Check sheet for the drawn part. Datum: minimum x, y, z corner. Units: mm. A direction names the side the tool comes from. Give positions to 0.01 mm unless a question says otherwise; leave off trailing zeros. Loops run counter-clockwise (first coordinate to the right, second up) from the corner with the lowest first, then second, coordinate; pieces in that order, holes last.
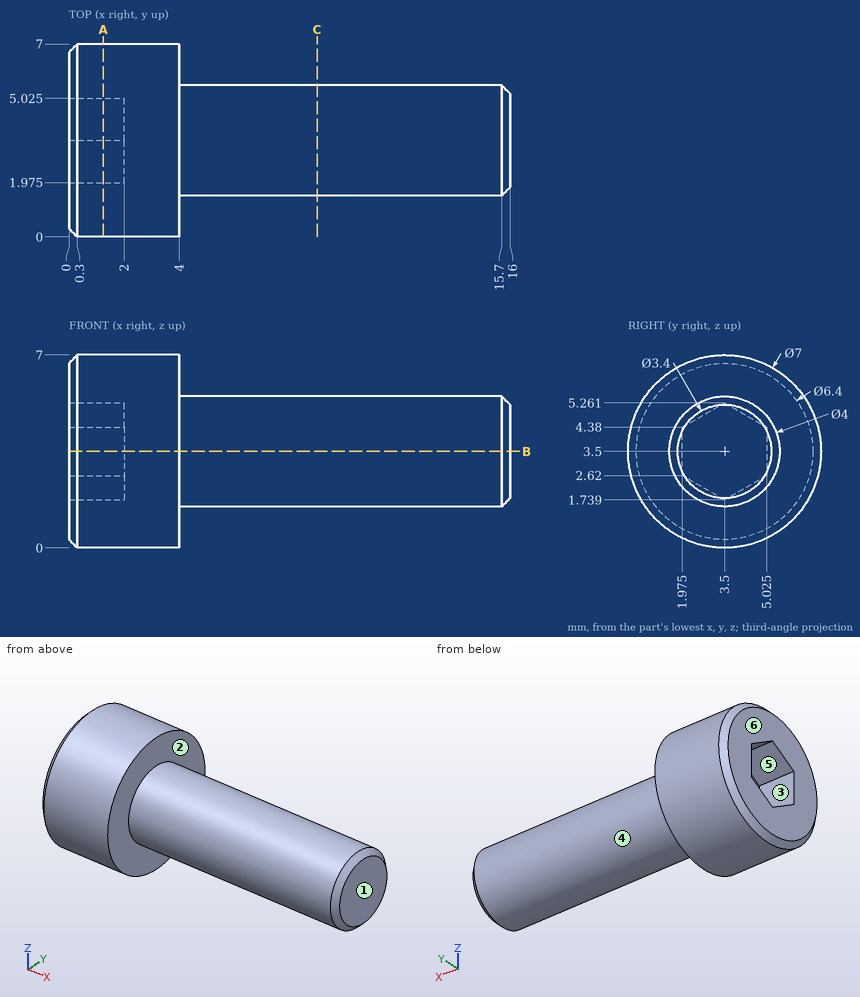
1) Sectioned sample at B-B on z = 3.5. Enter the section's corners in (x, y) (1 decimal).
2) Sectioned sample at A-A on x = 1.25. Enter the section's corners in (y, z) (1 decimal).
3) Depth check by flat-ended pin: P1, Ø1.5, axis at x = 11, y = 4, coming from the -Z side; P2, Ø3.5, axis at y = 2, z = 4.5, coming from the +X side; P3, Ø2, axis at x = 10.5, z = 1.5, coming from the +Y side; P4, Ø3, axis at x = 14, z = 5.5, coming from the -Y side. Enter the tip coordinate at first touch or a pass-through.
4) Scan lines: line 1 along X through (y, z) = (5.25, 1.75); line 2 along X through (y, z) = (2.5, 4); line 3 along Y through (x, z) = (13.75, 4.75). Record each from-to range of solid material in increasing order.
5) Sectioned sample at C-C on x = 9. Enter the section's corners in (y, z), plus the area to 3 significant figures.
6) Tool access check on the marked faces 1, 2 and 3. Record the directions out of +Z, -Z, +X, -X, +Y, -Y that give a thin tool (end or side, any length) a straight path to the whole face; none if there is none.
7) Mould release check, pull along Y, two halves, no side actions. Record for the marked faces 4, 5 and 6: +Y half, -Y half, draft (parallel to the pull), parting line (faces both ways), or undercut.
Determined:
1. outline: (0, 0.3) - (0.3, 0) - (4, 0) - (4, 1.5) - (15.7, 1.5) - (16, 1.8) - (16, 5.2) - (15.7, 5.5) - (4, 5.5) - (4, 7) - (0.3, 7) - (0, 6.7) - (0, 5) - (2, 5) - (2, 2) - (0, 2) - close
2. outline: circle Ø7 at (3.5, 3.5); hole (2, 2.6) - (3.5, 1.7) - (5, 2.6) - (5, 4.4) - (3.5, 5.3) - (2, 4.4) - close
3. P1: stops at z = 1.5
3. P2: stops at x = 16
3. P3: stops at y = 5.23
3. P4: stops at y = 1.56
4. line 1: x = 0 to 4
4. line 2: x = 2 to 16
4. line 3: y = 1.94 to 5.06
5. outline: circle Ø4 at (3.5, 3.5)
5. area: 12.6 mm2
6. face 1: +Z, -Z, +X, +Y, -Y
6. face 2: +X
6. face 3: -X
7. face 4: parting line
7. face 5: undercut
7. face 6: draft
